from build123d import *

# Parameters (mm, degrees)
F0_W      = 102.4
F0_H      = 147
F1_DEPTH  = 3
F2_W      = 3
F2_H      = 147
F3_DEPTH  = 10
F5_R      = 2.3
F6_DEPTH  = 102.401
F7_R      = 1.75
F8_DEPTH  = 3.001
F9_W      = 41.4
F9_H      = 60
F9_W_2    = 96.3999993775
F9_H_2    = 35.4163302109
F10_DEPTH = 12.5
F11_R     = 5


# Not quite as in the source:
# - a pattern or mirror of a feature is missing from the dataset's text; its kind, count and spacing are read off the source's solid
# - a feature names something its author has since deleted; it is built from what else it names


with BuildPart() as f1:
    # F0 (on Top) → F1 (new body)
    with BuildSketch(Plane.XY):
        with Locations((-12.3022546887, 26.2855888009)):
            Rectangle(F0_W, F0_H)
    extrude(amount=F1_DEPTH)

    # F2 (on face) → F3 (join)
    with BuildSketch(Plane.XY.offset(3)):
        with Locations((-62.0022546887, 26.2855888009)):
            Rectangle(F2_W, F2_H)
    f3 = extrude(amount=F3_DEPTH)

    # F3_copies: F3 across plane
    add(f3.mirror(Plane(origin=(-12.302255, 0, 0), x_dir=(0, 0, 1), z_dir=(1, 0, 0))))

    # F5 (on face) → F6 (cut, through all)
    with BuildSketch(Plane(origin=(-63.5022546887, 0, 0), x_dir=(0, -1, 0), z_dir=(-1, 0, 0))):
        with Locations((1.8144111991, 6.35)):
            Circle(F5_R)
        with Locations((-29.6755888009, 6.35)):
            Circle(F5_R)
        with Locations((-71.2855888009, 6.35)):
            Circle(F5_R)
    extrude(amount=-F6_DEPTH, mode=Mode.SUBTRACT)

    # F7 (on face) → F8 (cut, through all)
    with BuildSketch(Plane.XY.offset(3)):
        with Locations((26.5577453113, 9.1855888009)):
            Circle(F7_R)
        with Locations((-35.1622546887, 9.1855888009)):
            Circle(F7_R)
        with Locations((-35.1622546887, 85.7855888009)):
            Circle(F7_R)
        with Locations((26.5577453113, 85.7855888009)):
            Circle(F7_R)
    extrude(amount=-F8_DEPTH, mode=Mode.SUBTRACT)

    # F9 (on face) → F10 (cut, symmetric)
    with BuildSketch(Plane.XY.offset(3)):
        with Locations((-4.8022546887, 47.7176743746)):
            Rectangle(F9_W, F9_H)
        with Locations((-12.302255, -29.5062460937)):
            Rectangle(F9_W_2, F9_H_2)
        Polygon((-71.4376792312, -51.2489080429), (43.8891761005, -51.2489080429), (43.8891761005, -11.7980809882), (35.8977446887, -11.7980809882), (35.8977446887, -47.2144111991), (-60.5022546887, -47.2144111991), (-60.5022546887, -11.7980809882), (-71.4376792312, -11.7980809882), align=None)
    extrude(amount=F10_DEPTH, both=True, mode=Mode.SUBTRACT)

    # F11
    f11_edges = [f1.edges().sort_by_distance(p)[0] for p in [
        (-62.002255, 99.785589, 13),
        (-62.002255, -11.798081, 13),
        (15.897745, 17.717674, 1.5),
        (-25.502255, 17.717674, 1.5),
        (-25.502255, 77.717674, 1.5),
        (15.897745, 77.717674, 1.5),
        (37.397745, 99.785589, 13),
        (37.397745, -11.798081, 13),
    ]]
    fillet(f11_edges, radius=F11_R)


solid = f1.part
Source: CAD feature listing. Evaluate the final solid. Frame: model axes, mm. A direction names the side the tool comes from. Round coordinates to 2 decimals unless told otherwise and drop trailing zeros. Write each loop counter-clockwise with the first axis right and the second up, starting at its lowest first coordinate (ties: lowest second). Pieces come first, ordered by that corner, then holes. Notation, with made-up numbers: M 51.25,-8.75 L 104.25,-8.75 A8 cw 104.25,-4.75 Z; hole C 3.25,-39.75 d5. An arc over 180 degrees is marked long. One line per item, written item: value. Start each with the question number.
Item 1: Mould query, pull axis X, two halves, no side actions, for faces 4 (the flat face through (38.898, 43, 8)), 5 (the cylindrical face through (-36.45, 10.37, 1.52)), 6 (the cylindrical face through (-35.542, 84.077, 1.521)), 7 (the cylindrical face through (-62.023, -1.316, 4.105)). Classes: pulls with the +X half, pulls with the -X half, needs draft (parallel to the pull), parting line crosses it, or undercut.
Item 2: Set-up query: faces 1 (the cylindrical face through (-62.023, 73.583, 6.451)), 2 (the flat face through (-25.502, 47, 1)), 3 (the flat face through (-60.502, 43, 8)). Return all of +Z, -Z, +X, -X, +Y, -Y with unobstructed straight access to the full face (end or side cutting, diameter ignored); none if empty.
Item 3: Section query C-C (y = 90.5). Return the cut outline in (x, z), plus the area to 3 significant figures.
Item 4: Section query B-B (x = -17.5). Return the cut outline in (y, z), plus the area to 3 significant figures.
Item 5: Ray query, L1, parallel to X at y = 9.5, z = 1.5; L2, parallel to X at y = 25, z = 6.5; L3, parallel to X at y = 87, z = 0.5. Return the intervals inside material, ascending. Write a range as from..to.
Item 6: Section query D-D (x = -35). Return the cut outline in (y, z).
Item 7: Pin query (flat end, axial travel): pin 1 (4 mm diameter, centred on y = 71.29, z = 6.35, fed in from -X). Return the tip coordinate at first contact, or that it passes through.
Item 8: Section query A-A (z = 6.35). State how many separate pieces and enclosed holes the cut face has, plus the area to 3 significant figures.
Result set:
1. face 4: pulls with the +X half
1. face 5: undercut
1. face 6: undercut
1. face 7: needs draft
2. face 1: +X, -X
2. face 2: +Z, -Z
2. face 3: +Z, +Y, -Y
3. outline: M -63.5,0 L 38.9,0 L 38.9,13 L 35.9,13 L 35.9,3 L -60.5,3 L -60.5,13 L -63.5,13 Z
3. area: 367 mm²
4. outline: M -11.8,0 L 17.72,0 L 17.72,3 L -11.8,3 Z; M 77.72,0 L 99.79,0 L 99.79,3 L 77.72,3 Z
4. area: 155 mm²
5. L1: x = -63.5..-36.88, -33.44..24.84, 28.28..38.9
5. L2: x = -63.5..-60.5, 35.9..38.9
5. L3: x = -63.5..-36.42, -33.9..25.3, 27.82..38.9
6. outline: M -11.8,0 L 7.44,0 L 7.44,3 L -11.8,3 Z; M 10.93,0 L 84.04,0 L 84.04,3 L 10.93,3 Z; M 87.53,0 L 99.79,0 L 99.79,3 L 87.53,3 Z
7. pin 1: passes through
8. separate pieces: 8
8. enclosed holes: 0
8. area: 587 mm²
